Can you work these out from the model? Positions are in its coordinate system, mm. Face numbers are marked on the shaded views. A direction names the side the tool comes from. Give positions to 0.01 mm unless a question says otherwise; leave off trailing zeros. Write each loop counter-clockwise with the first axis right and the second up, starting at its lowest first coordinate (ties: lowest second). Pieces come first, ordered by that corner, then holes. Notation, with made-up numbers: (-10, 12.25) -> (26, 12.25) arc R27 cw to (26, 35.25) -> close; hole circle Ø4 at (48, 39.25). An arc over 180 degrees is marked (long way). One line per item, written item: value.
from build123d import *

# Parameters (mm, degrees)
F0_R     = 30
F1_DEPTH = 19.05
F0_R_2   = 3.175
F2_DEPTH = 19.05


with BuildPart() as f1:
    # F0 (on Front) → F1 (new body)
    with BuildSketch(Plane.XZ):
        Circle(F0_R)
        with BuildLine():
            ThreePointArc((-15.1925895519, 24.0154928425), (-9.4885710036, 26.7866700818), (-3.3120353789, 28.2239099951))
            ThreePointArc((-3.3120353789, 28.2239099951), (3.0733934985, 28.2508924844), (9.3036437218, 26.8514596858))
            ThreePointArc((9.3036437218, 26.8514596858), (15.0266347255, 24.119679156), (20.0013211104, 20.1867735808))
            ThreePointArc((20.0013211104, 20.1867735808), (24.0036666555, 15.2112675623), (26.7940435133, 9.4677297158))
            ThreePointArc((26.7940435133, 9.4677297158), (28.0087527775, 4.8029617543), (28.4175768454, 0))
            ThreePointArc((28.4175768454, 0), (28.376471618, -1.5279176275), (28.2532748509, -3.051415075))
            ThreePointArc((28.2532748509, -3.051415075), (26.8586892354, -9.2827520875), (24.1079820404, -15.0453938367))
            ThreePointArc((24.1079820404, -15.0453938367), (20.1712076487, -20.0170191526), (15.229936367, -23.9918259418))
            ThreePointArc((15.229936367, -23.9918259418), (9.4885710036, -26.7866700818), (3.2681183779, -28.2290289601))
            ThreePointArc((3.2681183779, -28.2290289601), (-3.0733934985, -28.2508924844), (-9.2618548354, -26.8659025303))
            ThreePointArc((-9.2618548354, -26.8659025303), (-15.0266347255, -24.119679156), (-20.0327050806, -20.1556295092))
            ThreePointArc((-20.0327050806, -20.1556295092), (-24.0036666555, -15.2112675623), (-26.7792804393, -9.509406549))
            ThreePointArc((-26.7792804393, -9.509406549), (-28.2264780188, -3.2900778739), (-28.2484930207, 3.095370062))
            ThreePointArc((-28.2484930207, 3.095370062), (-26.8586892354, 9.2827520875), (-24.1313616746, 15.0078665203))
            ThreePointArc((-24.1313616746, 15.0078665203), (-20.1712076487, 20.0170191526), (-15.1925895519, 24.0154928425))
        make_face(mode=Mode.SUBTRACT)
    extrude(amount=F1_DEPTH)

    # F0 (on Front) → F2 (join)
    with BuildSketch(Plane.XZ):
        with BuildLine():
            Line((-0.0086937801, 5.1407505785), (-3.3120353789, 28.2239099951))
            ThreePointArc((-3.3120353789, 28.2239099951), (-9.4885710036, 26.7866700818), (-15.1925895519, 24.0154928425))
            Line((-15.1925895519, 24.0154928425), (-4.0029845, 3.2254468194))
            ThreePointArc((-4.0029845, 3.2254468194), (-2.2227208053, 4.6353968885), (-0.0086937801, 5.1407505785))
        make_face()
        with BuildLine():
            ThreePointArc((20.0013211104, 20.1867735808), (15.0266347255, 24.119679156), (9.3036437218, 26.8514596858))
            Line((9.3036437218, 26.8514596858), (0.0259358557, 5.1406925043))
            ThreePointArc((0.0259358557, 5.1406925043), (2.2382554667, 4.6279157898), (4.0137801625, 3.2120026306))
            Line((4.0137801625, 3.2120026306), (20.0013211104, 20.1867735808))
        make_face()
        with BuildLine():
            ThreePointArc((28.4175768454, 0), (28.0087527775, 4.8029617543), (26.7940435133, 9.4677297158))
            Line((26.7940435133, 9.4677297158), (4.035325983, 3.1848918824))
            ThreePointArc((4.035325983, 3.1848918824), (4.8565433251, 1.6856390547), (5.1407579297, 0))
            ThreePointArc((5.1407579297, 0), (5.108918794, -0.5712625033), (5.0137957766, -1.135448811))
            Line((5.0137957766, -1.135448811), (28.2532748509, -3.051415075))
            ThreePointArc((28.2532748509, -3.051415075), (28.376471618, -1.5279176275), (28.4175768454, 0))
        make_face()
        with BuildLine():
            ThreePointArc((15.229936367, -23.9918259418), (20.1712076487, -20.0170191526), (24.1079820404, -15.0453938367))
            Line((24.1079820404, -15.0453938367), (5.0060333395, -1.1691972868))
            ThreePointArc((5.0060333395, -1.1691972868), (4.0138255819, -3.2119458729), (2.2383209081, -4.627884139))
            Line((2.2383209081, -4.627884139), (15.229936367, -23.9918259418))
        make_face()
        with BuildLine():
            Line((-2.2226552576, -4.6354283187), (-9.2618548354, -26.8659025303))
            ThreePointArc((-9.2618548354, -26.8659025303), (-3.0733934985, -28.2508924844), (3.2681183779, -28.2290289601))
            Line((3.2681183779, -28.2290289601), (2.2070954869, -4.6428570518))
            ThreePointArc((2.2070954869, -4.6428570518), (-0.0086210867, -5.1407507009), (-2.2226552576, -4.6354283187))
        make_face()
        with BuildLine():
            Line((-5.0099266804, -1.1524004289), (-26.7792804393, -9.509406549))
            ThreePointArc((-26.7792804393, -9.509406549), (-24.0036666555, -15.2112675623), (-20.0327050806, -20.1556295092))
            Line((-20.0327050806, -20.1556295092), (-2.2538302839, -4.6203507598))
            ThreePointArc((-2.2538302839, -4.6203507598), (-4.0245759011, -3.1984653989), (-5.0099266804, -1.1524004289))
        make_face()
        with BuildLine():
            Line((-4.024621129, 3.1984084886), (-24.1313616746, 15.0078665203))
            ThreePointArc((-24.1313616746, 15.0078665203), (-26.8586892354, 9.2827520875), (-28.2484930207, 3.095370062))
            Line((-28.2484930207, 3.095370062), (-5.0175758812, -1.1186261076))
            ThreePointArc((-5.0175758812, -1.1186261076), (-5.0099429756, 1.1523295852), (-4.024621129, 3.1984084886))
        make_face()
        with BuildLine():
            Line((0, 5.08), (-0.0086937801, 5.1407505785))
            ThreePointArc((-0.0086937801, 5.1407505785), (-2.2227208053, 4.6353968885), (-4.0029845, 3.2254468194))
            Line((-4.0029845, 3.2254468194), (-3.9717039309, 3.1673281934))
            Line((-3.9717039309, 3.1673281934), (-4.024621129, 3.1984084886))
            ThreePointArc((-4.024621129, 3.1984084886), (-5.0099429756, 1.1523295852), (-5.0175758812, -1.1186261076))
            Line((-5.0175758812, -1.1186261076), (-4.9526337939, -1.1304063445))
            Line((-4.9526337939, -1.1304063445), (-5.0099266804, -1.1524004289))
            ThreePointArc((-5.0099266804, -1.1524004289), (-4.0245759011, -3.1984653989), (-2.2538302839, -4.6203507598))
            Line((-2.2538302839, -4.6203507598), (-2.2041293947, -4.5769218489))
            Line((-2.2041293947, -4.5769218489), (-2.2226552576, -4.6354283187))
            ThreePointArc((-2.2226552576, -4.6354283187), (-0.0086210867, -5.1407507009), (2.2070954869, -4.6428570518))
            Line((2.2070954869, -4.6428570518), (2.2041293947, -4.5769218489))
            Line((2.2041293947, -4.5769218489), (2.2383209081, -4.627884139))
            ThreePointArc((2.2383209081, -4.627884139), (4.0138255819, -3.2119458729), (5.0060333395, -1.1691972868))
            Line((5.0060333395, -1.1691972868), (4.9526337939, -1.1304063445))
            Line((4.9526337939, -1.1304063445), (5.0137957766, -1.135448811))
            ThreePointArc((5.0137957766, -1.135448811), (5.108918794, -0.5712625033), (5.1407579297, 0))
            ThreePointArc((5.1407579297, 0), (4.8565433251, 1.6856390547), (4.035325983, 3.1848918824))
            Line((4.035325983, 3.1848918824), (3.9717039309, 3.1673281934))
            Line((3.9717039309, 3.1673281934), (4.0137801625, 3.2120026306))
            ThreePointArc((4.0137801625, 3.2120026306), (2.2382554667, 4.6279157898), (0.0259358557, 5.1406925043))
            Line((0.0259358557, 5.1406925043), (0, 5.08))
        make_face()
        Circle(F0_R_2, mode=Mode.SUBTRACT)
    extrude(amount=F2_DEPTH)


solid = f1.part
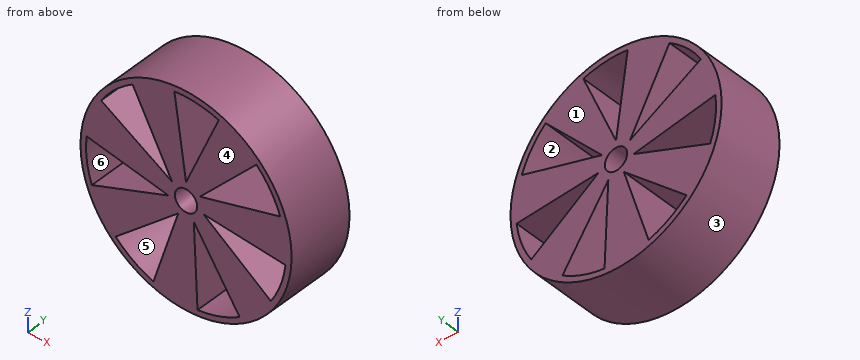
1) If we section it at B-B (x = -12.5): Write out the boundary of the cut face in (y, z).
Answer list:
outline: (-19.05, -27.27) -> (0, -27.27) -> (0, -25.52) -> (-19.05, -25.52) -> close; (-19.05, -13.57) -> (0, -13.57) -> (0, -4.03) -> (-19.05, -4.03) -> close; (-19.05, 0.24) -> (0, 0.24) -> (0, 8.18) -> (-19.05, 8.18) -> close; (-19.05, 19.01) -> (0, 19.01) -> (0, 27.27) -> (-19.05, 27.27) -> close
2) I need wall thicknesses on L1, parallel to Z at x = -12, y = -9.5; L2, parallel to Z at x = 13.5, y = -3.25; L3, parallel to X at y = -9.5, z = 11.5. Which ranges of each line are inside material? Lowest first, please.
Answer list:
L1: z = -27.5 to -25.76, -13.14 to -3.84, 0.15 to 7.88, 18.08 to 27.5
L2: z = -26.79 to -25.01, -21.41 to -7.34, -1.84 to 5.8, 13.28 to 26.79
L3: x = -27.71 to -18.16, -8.46 to -0.92, 2.74 to 11.82, 25.99 to 27.71
3) If we section it at C-C (z = -18): Write out the boundary of the cut face in (x, y), and give its area (3 significant figures).
Answer list:
outline: (-24, -19.05) -> (-17.57, -19.05) -> (-17.57, 0) -> (-24, 0) -> close; (-6.45, -19.05) -> (2.81, -19.05) -> (2.81, 0) -> (-6.45, 0) -> close; (11.21, -19.05) -> (24, -19.05) -> (24, 0) -> (11.21, 0) -> close
area: 543 mm^2
4) If we section it at D-D (y = -4.75): State how many separate pieces and enclosed holes the cut face has, and give its area (3 significant figures).
Answer list:
separate pieces: 1
enclosed holes: 8
area: 1,750 mm^2
5) Will these pins go through, and if not, where does the flat tip stop? pin 1 (2 mm diameter, centred on x = -10.5, y = -2.5, fed in from -Z); pin 2 (2 mm diameter, centred on x = 16, y = -15, fed in from -Z); pin 3 (8 mm diameter, centred on y = -3, z = -16, fed in from -X).
Answer list:
pin 1: stops at z = -28.46
pin 2: stops at z = -25.98
pin 3: stops at x = -27.5
6) If we section it at A-A (z = -10.5): Write out the boundary of the cut face in (x, y).
Answer list:
outline: (-28.1, -19.05) -> (-8.98, -19.05) -> (-8.98, 0) -> (-28.1, 0) -> close; (-4.08, -19.05) -> (2.47, -19.05) -> (2.47, 0) -> (-4.08, 0) -> close; (6.18, -19.05) -> (17.85, -19.05) -> (17.85, 0) -> (6.18, 0) -> close; (26.41, -19.05) -> (28.1, -19.05) -> (28.1, 0) -> (26.41, 0) -> close
7) We'd pull the mould along X, two halves only. Please class the marked faces 3, 4, 5 and 6: released by +X, released by -X, zero draft, split by the parting line, or undercut.
Answer list:
face 3: split by the parting line
face 4: zero draft
face 5: undercut
face 6: undercut
8) For the marked faces 1 and 2, which set-ups out of +Z, -Z, +X, -X, +Y, -Y let a thin tool reach every point of the face, with its end or its side?
Answer list:
face 1: +Z, -Z, +X, -X, +Y
face 2: +Y, -Y
